Read the model definition and answer for the solid it produces. Units are mm, in the model's axes. Coordinates: 2 decimals unless noted, no trailing zeros. Order: outer loops, then holes, each group sorted by start corner. A loop starts at its lowest first (then second) coordinate and runs counter-clockwise, first axis right, second up. Notation, with made-up numbers: M 55.25,3.5 L 63.25,3.5 A10 cw 63.25,21.5 Z; hole C -23.75,62.5 d7. An arc over 180 degrees is marked long. Use a Markdown table: item, result. Add a question column.
1) Find the intervals of material crossed by probe 1 along Z at (x, y) = (34, 0.3); probe 2 along X at (y, z) = (-1.2, 97); probe 3 along Z at (x, y) = (36, 0.35), in increasing order. Write a range as [from, to].
2) Find section B-B on y = -0.7. Count the separate pieces of the cut face and the enclosed holes in it, plus the area to 3 significant figures.
3) Find section A-A on x = 10. Write down the section's boundary in (y, z), plus the area to 4 significant figures.
4) This flat-tipped pin is pushed along its axis until it touches: pin 1 Ø5 at (x, z) = (16, 7.8) entering from +Y. Where does it stop, or does it pass through?
5) The mould has two halves that part along X. Classify faces 1 (the face through (15.71, 0.02, 124.43)), 2 (the face through (47, 0, 128)), 3 (the face through (25, 1.5, 66)): released by +X, released by -X, zero draft, split by the parting line, or undercut.
6) Find section C-C on x = 16. Write down the section's boundary in (y, z), plus the area to 3 significant figures.
7) Find section D-D on z = 61.8. Write down the section's boundary in (x, y).
from build123d import *

# Parameters (mm, degrees)
F0_W     = 50
F0_H     = 130
F0_R     = 2.25
F1_DEPTH = 1.5
F2_SIZE  = 5


with BuildPart() as f1:
    # F0 (on Front) → F1 (new body, symmetric)
    with BuildSketch(Plane.XZ):
        with Locations((25, 65)):
            Rectangle(F0_W, F0_H)
        with Locations((16, 7.8)):
            Circle(F0_R, mode=Mode.SUBTRACT)
        with Locations((16, 31.8)):
            Circle(F0_R, mode=Mode.SUBTRACT)
        with Locations((10, 61.8)):
            Circle(F0_R, mode=Mode.SUBTRACT)
        with Locations((34, 7.8)):
            Circle(F0_R, mode=Mode.SUBTRACT)
        with Locations((34, 31.8)):
            Circle(F0_R, mode=Mode.SUBTRACT)
        with Locations((40, 61.8)):
            Circle(F0_R, mode=Mode.SUBTRACT)
        with Locations((16, 98.2)):
            Circle(F0_R, mode=Mode.SUBTRACT)
        with Locations((16, 122.2)):
            Circle(F0_R, mode=Mode.SUBTRACT)
        with Locations((34, 98.2)):
            Circle(F0_R, mode=Mode.SUBTRACT)
        with Locations((34, 122.2)):
            Circle(F0_R, mode=Mode.SUBTRACT)
    extrude(amount=F1_DEPTH, both=True)

    # F2
    f2_edges = [f1.edges().sort_by_distance(p)[0] for p in [
        (0, 0, 0),
        (50, 0, 0),
        (0, 0, 130),
        (50, 0, 130),
    ]]
    chamfer(f2_edges, length=F2_SIZE)


solid = f1.part
Check result:
| question | item | result |
|---|---|---|
| 1 | probe 1 | z = [0, 5.55], [10.05, 29.55], [34.05, 95.95], [100.45, 119.95], [124.45, 130] |
| 1 | probe 2 | x = [0, 14.1], [17.9, 32.1], [35.9, 50] |
| 1 | probe 3 | z = [0, 6.77], [8.83, 30.77], [32.83, 97.17], [99.23, 121.17], [123.23, 130] |
| 2 | separate pieces | 1 |
| 2 | enclosed holes | 10 |
| 2 | area | 6,290 mm2 |
| 3 | outline | M -1.5,0 L 1.5,0 L 1.5,59.55 L -1.5,59.55 Z; M -1.5,64.05 L 1.5,64.05 L 1.5,130 L -1.5,130 Z |
| 3 | area | 376.5 mm2 |
| 4 | pin 1 | stops at y = 1.5 |
| 5 | face 1 | undercut |
| 5 | face 2 | released by +X |
| 5 | face 3 | zero draft |
| 6 | outline | M -1.5,0 L 1.5,0 L 1.5,5.55 L -1.5,5.55 Z; M -1.5,10.05 L 1.5,10.05 L 1.5,29.55 L -1.5,29.55 Z; M -1.5,34.05 L 1.5,34.05 L 1.5,95.95 L -1.5,95.95 Z; M -1.5,100.45 L 1.5,100.45 L 1.5,119.95 L -1.5,119.95 Z; M -1.5,124.45 L 1.5,124.45 L 1.5,130 L -1.5,130 Z |
| 6 | area | 336 mm2 |
| 7 | outline | M 0,-1.5 L 7.75,-1.5 L 7.75,1.5 L 0,1.5 Z; M 12.25,-1.5 L 37.75,-1.5 L 37.75,1.5 L 12.25,1.5 Z; M 42.25,-1.5 L 50,-1.5 L 50,1.5 L 42.25,1.5 Z |
